Part print with two shaded views. Sizes in mm from the minimum x, y, z corner. A direction names the side the tool comes from. Coordinates: 2 decimals unless noted, no trailing zeros. Loops run counter-clockwise (first coordinate to the right, second up) from the corner with the lowest first, then second, coordinate; pieces in that order, holes last. Notation, with made-up numbers: (9, 33) -> (63, 33) arc R9 ccw to (63, 49) -> close; hole circle Ø4 at (47, -24). An arc over 180 degrees is marked (long way). Write each question's results on one line, items separated by ' | '.
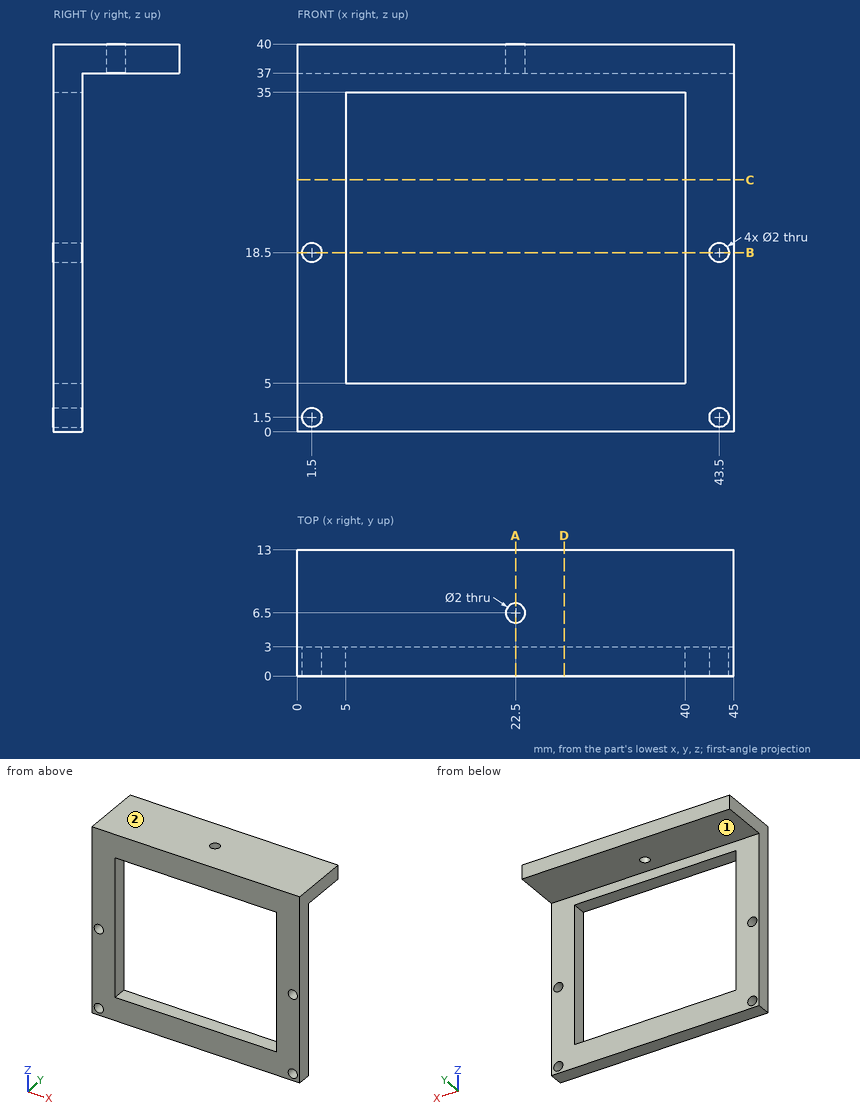
Q1. Drop flat-ended pins along their axis: pin 1 (3.5 mm diameter, centred on x = 16, y = 2, fed in from -Z); pin 2 (3 mm diameter, centred on x = 22.5, y = 6.5, fed in from -Z). Give the stop position or say it passes through.
Results are:
pin 1: z = 0 | pin 2: z = 37
Q2. Cut at C-C on z = 26. Write the cut outline in (x, y), and give its area (3 significant figures).
Results are:
outline: (0, 0) -> (5, 0) -> (5, 3) -> (0, 3) -> close; (40, 0) -> (45, 0) -> (45, 3) -> (40, 3) -> close | area: 30.0 mm^2
Q3. Cut at B-B on z = 18.5. Write the cut outline in (x, y).
Results are:
outline: (0, 0) -> (0.5, 0) -> (0.5, 3) -> (0, 3) -> close; (2.5, 0) -> (5, 0) -> (5, 3) -> (2.5, 3) -> close; (40, 0) -> (42.5, 0) -> (42.5, 3) -> (40, 3) -> close; (44.5, 0) -> (45, 0) -> (45, 3) -> (44.5, 3) -> close
Q4. Wall check: L1, parallel to X at y = 2.3, z = 18.5; L2, parallel to X at y = 1.3, z = 1.5; L3, parallel to Z at x = 33, y = 1.75. Give the ranges that are in metal, low to high. Write a range as from..to.
Results are:
L1: 0..0.5, 2.5..5, 40..42.5, 44.5..45 | L2: 0..0.5, 2.5..42.5, 44.5..45 | L3: 0..5, 35..40
Q5. Cut at A-A on x = 22.5. Write the cut outline in (y, z), and give its area (3 significant figures).
Results are:
outline: (0, 0) -> (3, 0) -> (3, 5) -> (0, 5) -> close; (0, 35) -> (3, 35) -> (3, 37) -> (5.5, 37) -> (5.5, 40) -> (0, 40) -> close; (7.5, 37) -> (13, 37) -> (13, 40) -> (7.5, 40) -> close | area: 54.0 mm^2
Q6. Cut at D-D on x = 27.5. Write the cut outline in (y, z).
Results are:
outline: (0, 0) -> (3, 0) -> (3, 5) -> (0, 5) -> close; (0, 35) -> (3, 35) -> (3, 37) -> (13, 37) -> (13, 40) -> (0, 40) -> close
Q7. Which spindle directions (+Z, -Z, +X, -X, +Y, -Y) get a long thin tool onto all of the face, cutting with end or side? Do the marked faces 1 and 2. Say none if no direction does.
Results are:
face 1: -Z, +X, -X, +Y | face 2: +Z, +X, -X, +Y, -Y
